Answer from the drawing. Dimensions are ordinates in mm from the lowest x, y and z of the part. A direction names the side the tool comes from. Coordinates: 2 decimals unless noted, no trailing zeros. Order: outer loops, then holes, each group sorted by start corner. A loop starts at its lowest first (then second) coordinate and runs counter-clockwise, first axis right, second up. Notation, with made-up numbers: M -6.5,-22 L 22.5,-22 A12 cw 22.5,-17 Z; hole C -34,61.5 d8. An arc over 180 degrees is marked long. One line per question, with ' | ' between items. Start each with the question number.
1) The mould has two halves that part along Y. Classify the marked faces 5, 6 and 7: +Y half, -Y half, draft (parallel to the pull), parting line (faces both ways), or undercut.
2) Consider probe 1 along Y at (x, z) = (11.25, 8.25); probe 2 along Y at (x, z) = (10.5, 11.25); probe 3 along Y at (x, z) = (13, 5.5) (1 decimal). Determine where each line is inside the solid, lowest interval first.
3) Find section A-A, the plane y = 27. Write down the section's boundary in (x, z), plus the area to 3 significant figures.
4) Find section B-B, the plane y = 15.5. Write down the section's boundary in (x, z) (1 decimal), plus the area to 4 significant figures.
5) A tool of negligible diameter and unlimited length cuts with its end or side. For the marked faces 1, 2, 3 and 4, from which of +Z, -Z, +X, -X, +Y, -Y can it reach the whole face along a straight path? Write none if from no direction.
6) Given P1, Ø6, axis at y = 24, z = 2, coming from the -X side; P2, Ø3, axis at x = 3, z = 3, coming from the -Y side; P3, Ø2, axis at x = 12, z = 13, coming from the +Y side, each flat-ended and moving along its own axis, determine where each tip first touches the part or whether it passes through.
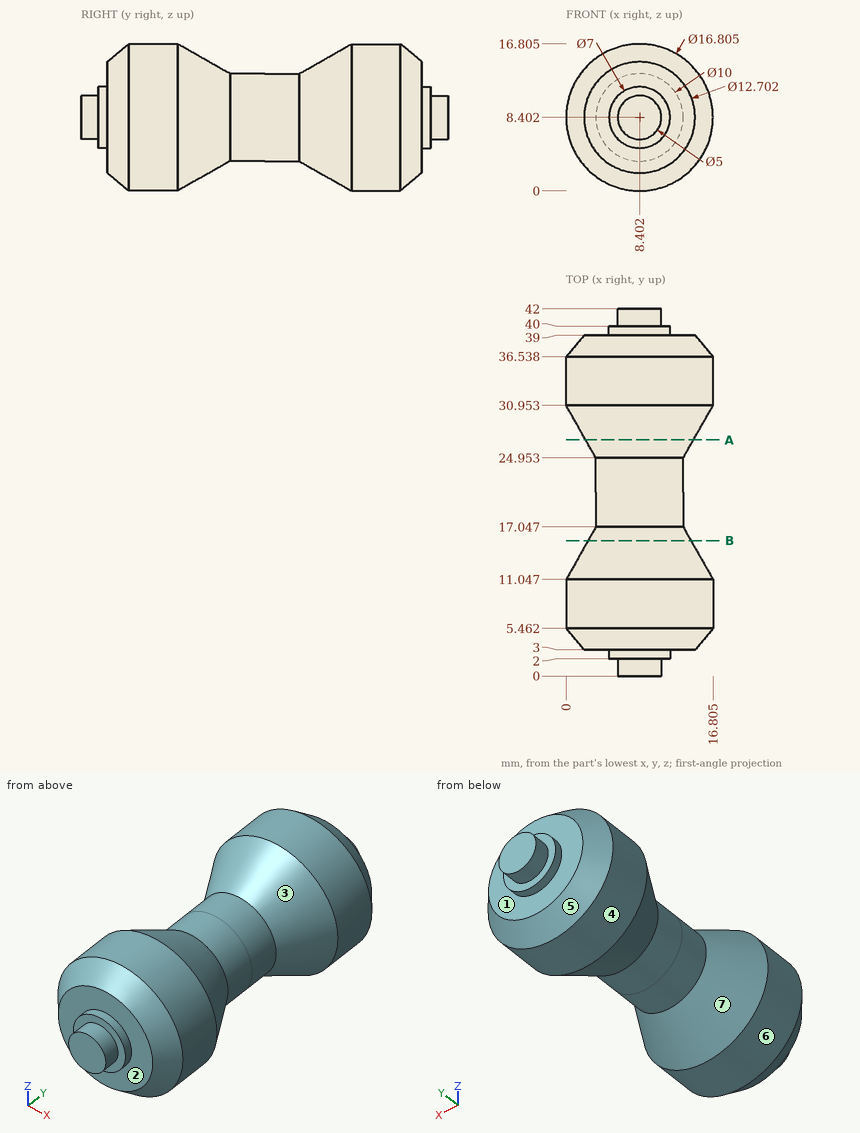
Report:
1) face 5: +Y half | face 6: draft | face 7: undercut
2) probe 1: y = 2 to 40 | probe 2: y = 3 to 39 | probe 3: y = 3 to 16.3, 25.7 to 39
3) outline: C 8.4,8.4 d12.32 | area: 119 mm^2
4) outline: C 8.4,8.4 d11.8 | area: 108.5 mm^2
5) face 1: +Y | face 2: -Y | face 3: none | face 4: +Y, -Y
6) P1: stops at x = 4.66 | P2: stops at y = 3 | P3: stops at y = 39
